from build123d import *

# Parameters (mm, degrees)
F1_DEPTH      = 12.7
F4_DEPTH      = 16.8285
F4_DEPTH_BACK = 16.8285
F5_R          = 2.54
F6_W          = 5.334
F6_H          = 2.032
F8_W          = 7.62
F8_H          = 2.54
F9_DEPTH      = 12.701
F9_DEPTH_BACK = 12.701
F10_W         = 2.032
F10_H         = 5.715
F13_DEPTH     = 33.656
F14_R         = 1.90499


# Not quite as in the source:
# - a fillet or chamfer is up to 0.001 mm smaller than in the source, because OpenCascade refuses the exact size


with BuildPart() as f1:
    # F0 (on Front) → F1 (new body, symmetric)
    with BuildSketch(Plane.XZ):
        with BuildLine():
            Line((0, 16.8275), (0, -16.8275))
            Line((0, -16.8275), (35.2425, -16.8275))
            ThreePointArc((35.2425, -16.8275), (18.415, 0), (35.2425, 16.8275))
            Line((35.2425, 16.8275), (0, 16.8275))
        make_face()
    extrude(amount=F1_DEPTH, both=True)

    # F3 (on Top) → F4 (cut, two sides)
    with BuildSketch(Plane.XY) as f4_sk:
        with BuildLine():
            Line((0, 10.795), (0, -10.795))
            ThreePointArc((0, -10.795), (10.795, 0), (0, 10.795))
        make_face()
    extrude(amount=-F4_DEPTH, mode=Mode.SUBTRACT)
    extrude(f4_sk.sketch, amount=F4_DEPTH_BACK, mode=Mode.SUBTRACT)

    # F5
    f5_edges = [f1.edges().sort_by_distance(p)[0] for p in [
        (35.2425, 0, 16.8275),
    ]]
    fillet(f5_edges, radius=F5_R)

    # F6 (on offset) → F7 (revolve, cut)
    with BuildSketch(Plane.YZ.offset(32.7025)):
        with Locations((7.493, 19.7485)):
            Rectangle(F6_W, F6_H)
        with Locations((-7.493, 19.7485)):
            Rectangle(F6_W, F6_H)
    revolve(axis=Axis((35.2425, 0, 0), (0, -1, 0)), mode=Mode.SUBTRACT)

    # F8 (on Front) → F9 (cut, two sides)
    with BuildSketch(Plane.XZ) as f9_sk:
        with Locations((31.4325, -15.5575)):
            Rectangle(F8_W, F8_H)
    extrude(amount=F9_DEPTH, mode=Mode.SUBTRACT)
    extrude(f9_sk.sketch, amount=-F9_DEPTH_BACK, mode=Mode.SUBTRACT)

    # F10 (on Right) → F11 (revolve, cut)
    with BuildSketch(Plane.YZ):
        with Locations((-15.621, 11.43)):
            Rectangle(F10_W, F10_H)
        with Locations((-15.621, -11.43)):
            Rectangle(F10_W, F10_H)
    revolve(axis=Axis((0, 0, 0), (0, 0, 1)), mode=Mode.SUBTRACT)

    # F12 (on face) → F13 (cut, through all)
    with BuildSketch(Plane.XY.offset(16.8275)):
        Polygon((5.6866191131, 9.17575), (0, 12.7), (0, 9.17575), align=None)
        Polygon((5.6866191131, -9.17575), (0, -9.17575), (0, -12.7), align=None)
    extrude(amount=-F13_DEPTH, mode=Mode.SUBTRACT)

    # F14 (radius 1.905 in the source; OpenCascade refuses exactly that, so slightly less here)
    f14_edges = [f1.edges().sort_by_distance(p)[0] for p in [
        (0, 12.7, 0),
        (0, -12.7, 0),
    ]]
    fillet(f14_edges, radius=F14_R)


solid = f1.part
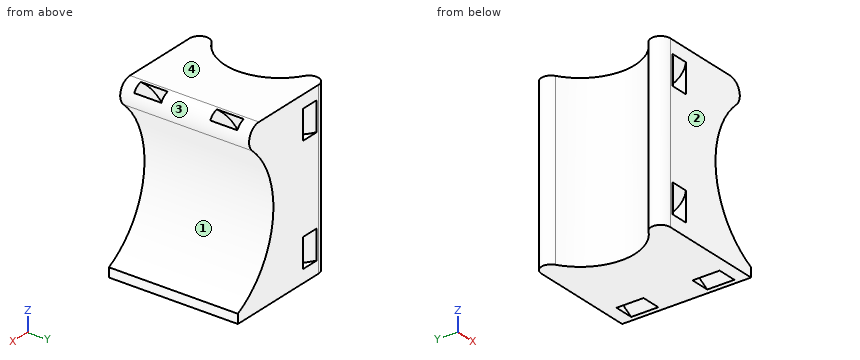
Design review of the part built by this model. Coordinates are the model's own, in mm. Face numbers are marked on the shaded views. Give positions to 0.01 mm unless a question says otherwise; leave off trailing zeros. Loops run counter-clockwise (first coordinate to the right, second up) from the corner with the lowest first, then second, coordinate; pieces in that order, holes last. Notation, with made-up numbers: M 17.25,42 L 27.25,42 A23 cw 27.25,54 Z; hole C -38.5,86 d10. An arc over 180 degrees is marked long. Answer as a JSON object with one key per item and string values.
Item 1: We need section D-D (x = 13.5). State the section outline as (y, z) points.
Output values:
{"outline": "M -12.7,-16.83 L 12.7,-16.83 L 12.7,16.83 L -12.7,16.83 Z; hole M -9.72,-14.29 L -5.57,-14.29 L -5.57,-8.57 L -9.72,-8.57 Z; hole M -9.72,8.57 L -5.57,8.57 L -5.57,14.29 L -9.72,14.29 Z; hole M 5.57,-14.29 L 9.72,-14.29 L 9.72,-8.57 L 5.57,-8.57 Z; hole M 5.57,8.57 L 9.72,8.57 L 9.72,14.29 L 5.57,14.29 Z"}
Item 2: We need section B-B (y = 7.25). State the section outline as (x, z) points (1 decimal).
Output values:
{"outline": "M 8,-16.8 L 22.8,-16.8 A20.9 cw 22.7,16.8 A2.5 ccw 22.2,16.8 L 8,16.8 Z; M 23.9,12.4 A2.5 ccw 24.4,15.5 A18.9 ccw 26.6,-16.8 L 27.6,-16.8 L 27.6,-15 A16.8 cw Z; hole M 12.7,-14.3 L 15,-14.3 L 15,-8.6 L 12.7,-8.6 Z; hole M 12.7,8.6 L 15,8.6 L 15,14.3 L 12.7,14.3 Z"}
Item 3: We need section C-C (x = 20.5). State the section outline as (y, z) points.
Output values:
{"outline": "M -12.7,-16.83 L 12.7,-16.83 L 12.7,-8.11 L -12.7,-8.11 Z; M -12.7,8.11 L 12.7,8.11 L 12.7,16.83 L -12.7,16.83 Z; hole M -10.16,-14.84 L -4.83,-14.84 L -4.83,-11.83 L -10.16,-11.83 Z; hole M -10.16,11.83 L -4.83,11.83 L -4.83,14.84 L -10.16,14.84 Z; hole M 4.83,-14.84 L 10.16,-14.84 L 10.16,-11.83 L 4.83,-11.83 Z; hole M 4.83,11.83 L 10.16,11.83 L 10.16,14.84 L 4.83,14.84 Z"}
Item 4: For P1, Ø2, axis at x = 9.5, y = 4, coming from the -Z side; P2, Ø10, axis at y = -9, z = 9.5, coming from the +X side; P3, Ø1, axis at y = -9.5, z = 1.5, coming from the +X side; P4, Ø6, axis at y = -0.5, z = 0.5, coming from the +X side, all flat-tipped, find the tip position at first contact; note any pin that passes through.
Output values:
{"P1": "stops at z = -16.83", "P2": "stops at x = 24.71", "P3": "stops at x = 18.53", "P4": "stops at x = 18.78"}
Item 5: We need section A-A (z = 9). Count the separate pieces of the cut face and the enclosed holes in it, and give its area (3 significant figures).
Output values:
{"separate pieces": "2", "enclosed holes": "2", "area": "243 mm2"}
Item 6: Wall thickness on line 1 along Y through (x, z) = (18, 11); line 2 along Z through (x, y) = (21, 7.5); line 3 along X through (y, z) = (-8.75, -14): over which ranges is each line inside the solid? List them lowest first.
Output values:
{"line 1": "y = -12.7 to -10.16, -4.83 to 4.83, 10.16 to 12.7", "line 2": "z = -16.83 to -15.32, -12.43 to -8.96, 8.96 to 12.43, 15.32 to 16.83", "line 3": "x = 6.32 to 11.69, 14.15 to 19.7, 22.54 to 25.91"}
Item 7: Mouldability with a two-part tool opening along Z and no side actions: class the marked faces 1, 2, 3 and 4 as pulls with the +Z half, pulls with the -Z half, needs draft (parallel to the pull), parting line crosses it, or undercut.
Output values:
{"face 1": "undercut", "face 2": "needs draft", "face 3": "undercut", "face 4": "pulls with the +Z half"}
